from build123d import *

# Parameters (mm, degrees)
SKETCH1_R           = 4.9
SKETCH1_R_2         = 2.6
SKETCH1_R_3         = 1.6
SKETCH1_R_4         = 11.25
BOSS_EXTRUDE1_DEPTH = 3.125
FILLET1_R           = 8
CUT_EXTRUDE1_REACH  = 5.125
SKETCH3_R           = 1.6


with BuildPart() as part:
    # Sketch1 → Boss-Extrude1 (new body)
    with BuildSketch(Plane(origin=(0, 0, 0), x_dir=(1, 0, 0), z_dir=(0, 1, 0))):
        with BuildLine():
            Line((-27.5, 86.48), (-21.5, 86.48))
            Line((-21.5, 86.48), (-21.5, 3.35))
            Line((-21.5, 3.35), (-18.15, 0))
            Line((-18.15, 0), (18.15, 0))
            Line((18.15, 0), (21.5, 3.35))
            Line((21.5, 3.35), (21.5, 75.517491819))
            ThreePointArc((21.5, 75.517491819), (19.195241391, 81.531952951), (13.461390508, 84.465996068))
            ThreePointArc((13.461390508, 84.465996068), (-3.952756456, 90.933879006), (-16.17349063, 104.924578791))
            ThreePointArc((-16.17349063, 104.924578791), (-38.32234149, 105.825820091), (-27.5, 86.48))
        make_face()
        with Locations((-27.5, 99.18)):
            Circle(SKETCH1_R, mode=Mode.SUBTRACT)
        with Locations((10, 77)):
            Circle(SKETCH1_R_2, mode=Mode.SUBTRACT)
        with Locations((-10, 77)):
            Circle(SKETCH1_R_2, mode=Mode.SUBTRACT)
        with Locations((10, 10)):
            Circle(SKETCH1_R_3, mode=Mode.SUBTRACT)
        with Locations((-10, 10)):
            Circle(SKETCH1_R_3, mode=Mode.SUBTRACT)
        with Locations((-20.355290419, 95.055)):
            Circle(SKETCH1_R_3, mode=Mode.SUBTRACT)
        with Locations((-34.644709581, 95.055)):
            Circle(SKETCH1_R_3, mode=Mode.SUBTRACT)
        with Locations((-27.5, 107.43)):
            Circle(SKETCH1_R_3, mode=Mode.SUBTRACT)
        with Locations((0, 42)):
            Circle(SKETCH1_R_4, mode=Mode.SUBTRACT)
        with Locations((-15.5, 26.5)):
            Circle(SKETCH1_R_3, mode=Mode.SUBTRACT)
        with Locations((-15.5, 57.5)):
            Circle(SKETCH1_R_3, mode=Mode.SUBTRACT)
        with Locations((15.5, 57.5)):
            Circle(SKETCH1_R_3, mode=Mode.SUBTRACT)
        with Locations((15.5, 26.5)):
            Circle(SKETCH1_R_3, mode=Mode.SUBTRACT)
    extrude(amount=BOSS_EXTRUDE1_DEPTH)

    # Fillet1
    fillet1_edges = [part.edges().sort_by_distance(p)[0] for p in [
        (-21.5, 1.5625, -86.48),
    ]]
    fillet(fillet1_edges, radius=FILLET1_R)

    # Sketch3 → Cut-Extrude1 (cut, up to next)
    with BuildSketch(Plane(origin=(0, 3.125, 0), x_dir=(1, 0, 0), z_dir=(0, 1, 0)), mode=Mode.PRIVATE) as cut_extrude1_sk1:
        with Locations((-27.5, 89.653720558)):
            Circle(SKETCH3_R)
    cut_extrude1_tool1 = extrude(cut_extrude1_sk1.sketch, amount=-CUT_EXTRUDE1_REACH, mode=Mode.PRIVATE) & part.part
    add(cut_extrude1_tool1.solids().sort_by_distance((-27.5, 3.125, -89.653721))[0], mode=Mode.SUBTRACT)
    # Sketch3 → Cut-Extrude1 (cut, up to next)
    with BuildSketch(Plane(origin=(0, 3.125, 0), x_dir=(1, 0, 0), z_dir=(0, 1, 0)), mode=Mode.PRIVATE) as cut_extrude1_sk2:
        with Locations((-35.75, 103.943139721)):
            Circle(SKETCH3_R)
    cut_extrude1_tool2 = extrude(cut_extrude1_sk2.sketch, amount=-CUT_EXTRUDE1_REACH, mode=Mode.PRIVATE) & part.part
    add(cut_extrude1_tool2.solids().sort_by_distance((-35.75, 3.125, -103.94314))[0], mode=Mode.SUBTRACT)
    # Sketch3 → Cut-Extrude1 (cut, up to next)
    with BuildSketch(Plane(origin=(0, 3.125, 0), x_dir=(1, 0, 0), z_dir=(0, 1, 0)), mode=Mode.PRIVATE) as cut_extrude1_sk3:
        with Locations((-19.25, 103.943139721)):
            Circle(SKETCH3_R)
    cut_extrude1_tool3 = extrude(cut_extrude1_sk3.sketch, amount=-CUT_EXTRUDE1_REACH, mode=Mode.PRIVATE) & part.part
    add(cut_extrude1_tool3.solids().sort_by_distance((-19.25, 3.125, -103.94314))[0], mode=Mode.SUBTRACT)


solid = part.part
Read the model definition and answer for the solid it produces. Units are mm, in the model's axes. A direction names the side the tool comes from. Give positions to 0.01 mm unless a question says otherwise; leave off trailing zeros. Write each loop counter-clockwise with the first axis right and the second up, starting at its lowest first coordinate (ties: lowest second). Pieces come first, ordered by that corner, then holes. Notation, with made-up numbers: (62.25, -39.5) - (107.25, -39.5) arc R26 cw to (107.25, -22.5) - close; hole circle Ø8 at (24.25, 60.5). An arc over 180 degrees is marked (long way). Use CSV: the item, a comma, the result in double quotes. Start each with the question number.
(1) Consider line 1 along X through (y, z) = (1.75, -26.5); line 2 along X through (y, z) = (0.85, -77); line 3 along Z through (x, y) = (-28.5, 2.3). Determine where each line is inside the solid, lowest interval first.
(2) Determine the mould class of faces 3 (the cylindrical face through (-16.68, 1.54, -27.58)), 4 (the cylindrical face through (9.662, 1.541, -79.578)), 5 (the cylindrical face through (-3.74, 1.54, -90.79)), 6 (the flat face through (-3, 3.125, -57)) for opening direction X: +X half, -X half, draft (parallel to the pull), parting line (faces both ways), or undercut.
(3) Given P1, Ø1, axis at y = 2, z = -64, coming from the -X side; P2, Ø4, axis at x = -20.36, z = -95.06, coming from the -Y side; P3, Ø3, axis at x = -35.75, z = -103.94, coming from the -Y side; P4, Ø1.5, axis at x = 7, y = 1.5, coming from the -Z side, each flat-ended and moving along its own axis, determine where each tip first touches the part or whether it passes through.
(4) Find section C-C (z = -77). Give the vertices of the cut face in (x, y) (3 decimals).
(5) For faces 1 (the cylindrical face through (-37.78, 1.54, -106.64)), 2 (the flat face through (-21.5, 2, -41)), determine the directions among +Z, -Z, +X, -X, +Y, -Y from which every point of the face is accessible in a straight line to the end or side of a thin tool.
(6) Find section D-D (y = 1.05). Count the separate pieces of the cut face and the enclosed holes in it, plus the area to 3 significant figures.
(7) Find section B-B (x = -9.5). Give the vertices of the cut face in (y, z) (3 decimals), plus the area to 3 significant figures.
(8) Find section A-A (z = -42). Give the vertices of the cut face in (x, y) (3 decimals).
Findings below:
1,line 1,"-21.5 to -17.1, -13.9 to 13.9, 17.1 to 21.5"
1,line 2,"-21.5 to -12.6, -7.4 to 7.4, 12.6 to 21.38"
1,line 3,"-111.84 to -108.68, -106.18 to -103.98, -94.38 to -90.9, -88.4 to -86.51"
2,face 3,"undercut"
2,face 4,"undercut"
2,face 5,"+X half"
2,face 6,"draft"
3,P1,"x = -21.5"
3,P2,"y = 0"
3,P3,"through"
3,P4,"z = -85.96"
4,outline,"(-21.5, 0) - (-12.6, 0) - (-12.6, 3.125) - (-21.5, 3.125) - close; (-7.4, 0) - (7.4, 0) - (7.4, 3.125) - (-7.4, 3.125) - close; (12.6, 0) - (21.377, 0) - (21.377, 3.125) - (12.6, 3.125) - close"
5,face 1,"+Y, -Y"
5,face 2,"+Z, -X, +Y, -Y"
6,separate pieces,"1"
6,enclosed holes,"16"
6,area,"3,730 mm2"
7,outline,"(0, -95.611) - (3.125, -95.611) - (3.125, -79.551) - (0, -79.551) - close; (0, -74.449) - (3.125, -74.449) - (3.125, -48.026) - (0, -48.026) - close; (0, -35.974) - (3.125, -35.974) - (3.125, -11.52) - (0, -11.52) - close; (0, -8.48) - (3.125, -8.48) - (3.125, 0) - (0, 0) - close"
7,area,"236 mm2"
8,outline,"(-21.5, 0) - (-11.25, 0) - (-11.25, 3.125) - (-21.5, 3.125) - close; (11.25, 0) - (21.5, 0) - (21.5, 3.125) - (11.25, 3.125) - close"
